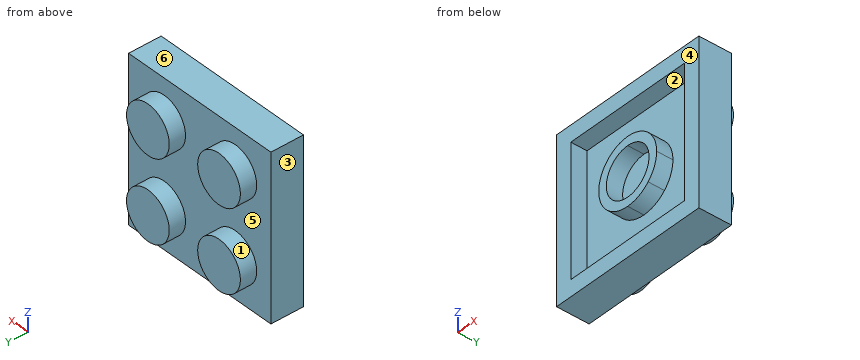
from build123d import *

# Parameters (mm, degrees)
SKETCH1_W           = 2.5
SKETCH1_H           = 1
BOSS_EXTRUDE1_DEPTH = 1
SKETCH1_4_W         = 2.5
SKETCH1_4_H         = 1
BOSS_EXTRUDE3_DEPTH = 1
SKETCH2_R           = 1.5
BOSS_EXTRUDE4_DEPTH = 1


with BuildPart() as part:
    # Sketch1 → Boss-Extrude1 (new body)
    with BuildSketch(Plane(origin=(0, 0, 0), x_dir=(1, 0, 0), z_dir=(0, 1, 0))):
        Polygon((5, 9), (5, 10), (0, 10), (0, 0), (5, 0), (5, 1), (1, 1), (1, 9), align=None)
        with BuildLine():
            Line((5, 7.035533906), (5, 9))
            Line((5, 9), (1, 9))
            Line((1, 9), (1, 1))
            Line((1, 1), (5, 1))
            Line((5, 1), (5, 2.964466094))
            ThreePointArc((5, 2.964466094), (2.964466094, 5), (5, 7.035533906))
        make_face()
        with BuildLine():
            ThreePointArc((6.439339828, 6.439339828), (5.778965102, 6.880588113), (5, 7.035533906))
            Line((5, 7.035533906), (5, 6.5))
            ThreePointArc((5, 6.5), (6.060660172, 6.060660172), (6.5, 5))
            ThreePointArc((6.5, 5), (6.060660172, 3.939339828), (5, 3.5))
            Line((5, 3.5), (5, 2.964466094))
            ThreePointArc((5, 2.964466094), (6.439339828, 3.560660172), (7.035533906, 5))
            ThreePointArc((7.035533906, 5), (6.880588113, 5.778965102), (6.439339828, 6.439339828))
        make_face()
        with BuildLine():
            Line((5, 6.5), (5, 7.035533906))
            ThreePointArc((5, 7.035533906), (2.964466094, 5), (5, 2.964466094))
            Line((5, 2.964466094), (5, 3.5))
            ThreePointArc((5, 3.5), (3.5, 5), (5, 6.5))
        make_face()
        with BuildLine():
            ThreePointArc((6.5, 5), (6.060660172, 6.060660172), (5, 6.5))
            Line((5, 6.5), (5, 3.5))
            ThreePointArc((5, 3.5), (6.060660172, 3.939339828), (6.5, 5))
        make_face()
        with BuildLine():
            Line((5, 3.5), (5, 6.5))
            ThreePointArc((5, 6.5), (3.5, 5), (5, 3.5))
        make_face()
        with BuildLine():
            Line((7.5, 9), (5, 9))
            Line((5, 9), (5, 7.035533906))
            ThreePointArc((5, 7.035533906), (5.778965102, 6.880588113), (6.439339828, 6.439339828))
            ThreePointArc((6.439339828, 6.439339828), (6.114180701, 8.074025149), (7.5, 9))
        make_face()
        with Locations((6.25, 9.5)):
            Rectangle(SKETCH1_W, SKETCH1_H)
        Polygon((10, 10), (7.5, 10), (7.5, 9), (9, 9), (9, 7.5), (10, 7.5), align=None)
        with BuildLine():
            Line((9, 9), (7.5, 9))
            ThreePointArc((7.5, 9), (8.560660172, 8.560660172), (9, 7.5))
            Line((9, 7.5), (9, 9))
        make_face()
        with BuildLine():
            ThreePointArc((9, 7.5), (8.560660172, 8.560660172), (7.5, 9))
            Line((7.5, 9), (7.5, 7.5))
            Line((7.5, 7.5), (9, 7.5))
        make_face()
        with BuildLine():
            Line((7.5, 7.5), (7.5, 9))
            ThreePointArc((7.5, 9), (6.114180701, 8.074025149), (6.439339828, 6.439339828))
            ThreePointArc((6.439339828, 6.439339828), (8.074025149, 6.114180701), (9, 7.5))
            Line((9, 7.5), (7.5, 7.5))
        make_face()
        with BuildLine():
            ThreePointArc((9, 7.5), (8.074025149, 6.114180701), (6.439339828, 6.439339828))
            ThreePointArc((6.439339828, 6.439339828), (6.880588113, 5.778965102), (7.035533906, 5))
            ThreePointArc((7.035533906, 5), (6.439339828, 3.560660172), (5, 2.964466094))
            Line((5, 2.964466094), (5, 1))
            Line((5, 1), (9, 1))
            Line((9, 1), (9, 7.5))
        make_face()
        Polygon((10, 7.5), (9, 7.5), (9, 1), (5, 1), (5, 0), (10, 0), align=None)
    extrude(amount=BOSS_EXTRUDE1_DEPTH)

    # Sketch1_4 → Boss-Extrude3 (add)
    with BuildSketch(Plane(origin=(0, 0, 0), x_dir=(1, 0, 0), z_dir=(0, 1, 0))):
        with BuildLine():
            ThreePointArc((6.439339828, 6.439339828), (5.778965102, 6.880588113), (5, 7.035533906))
            Line((5, 7.035533906), (5, 6.5))
            ThreePointArc((5, 6.5), (6.060660172, 6.060660172), (6.5, 5))
            ThreePointArc((6.5, 5), (6.060660172, 3.939339828), (5, 3.5))
            Line((5, 3.5), (5, 2.964466094))
            ThreePointArc((5, 2.964466094), (6.439339828, 3.560660172), (7.035533906, 5))
            ThreePointArc((7.035533906, 5), (6.880588113, 5.778965102), (6.439339828, 6.439339828))
        make_face()
        with BuildLine():
            Line((5, 6.5), (5, 7.035533906))
            ThreePointArc((5, 7.035533906), (2.964466094, 5), (5, 2.964466094))
            Line((5, 2.964466094), (5, 3.5))
            ThreePointArc((5, 3.5), (3.5, 5), (5, 6.5))
        make_face()
        Polygon((5, 9), (5, 10), (0, 10), (0, 0), (5, 0), (5, 1), (1, 1), (1, 9), align=None)
        Polygon((10, 7.5), (9, 7.5), (9, 1), (5, 1), (5, 0), (10, 0), align=None)
        Polygon((10, 10), (7.5, 10), (7.5, 9), (9, 9), (9, 7.5), (10, 7.5), align=None)
        with Locations((6.25, 9.5)):
            Rectangle(SKETCH1_4_W, SKETCH1_4_H)
    extrude(amount=-BOSS_EXTRUDE3_DEPTH)

    # Sketch2 → Boss-Extrude4 (add)
    with BuildSketch(Plane(origin=(0, 1, 0), x_dir=(1, 0, 0), z_dir=(0, 1, 0))):
        with Locations((7.5, 2.5)):
            Circle(SKETCH2_R)
        with Locations((2.5, 2.5)):
            Circle(SKETCH2_R)
        with Locations((2.5, 7.5)):
            Circle(SKETCH2_R)
        with Locations((7.5, 7.5)):
            Circle(SKETCH2_R)
    extrude(amount=BOSS_EXTRUDE4_DEPTH)


solid = part.part
Model file for the job. Use its own axes, mm. Face numbers are marked on the shaded views. A direction names the side the tool comes from. Give positions to 0.01 mm unless a question says otherwise; leave off trailing zeros. Loops run counter-clockwise (first coordinate to the right, second up) from the corner with the lowest first, then second, coordinate; pieces in that order, holes last.
1) Saw through at D-D (x = 9.5). Write the cut outline in (y, z), plus the area to 3 significant figures.
2) Pull direction Z, two halves, no side cores. Call the marked faces 4, 5 and 6: +Z half, -Z half, draft (parallel to the pull), parting line (faces both ways), or undercut.
3) Saw through at B-B (x = 7.5). Write the cut outline in (y, z).
4) Saw through at A-A (y = -0.2). Write the cut outline in (x, z), plus the area to 3 significant figures.
5) Saw through at C-C (z = -7.5). Write the cut outline in (x, y), plus the area to 3 significant figures.
6) Flat gauge pin, fed straight in: pin 1 Ø1 at (x, z) = (4.5, -5.5) entering from -Y. Where does the tip first touch, or does it go through?
7) Tool access for the marked faces 1, 2 and 3: list every direction of +Z, -Z, +X, -X, +Y, -Y with a clear straight run to the whole face (end or side of a thin tool).
8) Wall check: line 1 (Z direction, x = 5, y = -0.8); line 2 (Z direction, x = 7.5, y = 1.7); line 3 (Z direction, x = 8, y = -0.25). Give the ranges that are in metal, low to high.
Answer block:
1. outline: (-1, -10) - (1, -10) - (1, 0) - (-1, 0) - close
1. area: 20.0 mm2
2. face 4: draft
2. face 5: undercut
2. face 6: +Z half
3. outline: (-1, -10) - (1, -10) - (1, -9) - (2, -9) - (2, -6) - (1, -6) - (1, -4) - (2, -4) - (2, -1) - (1, -1) - (1, 0) - (-1, 0) - (-1, -1) - (0, -1) - (0, -9) - (-1, -9) - close
4. outline: (0, -10) - (10, -10) - (10, 0) - (0, 0) - close; circle Ø4.07 at (5, -5); hole (1, -9) - (9, -9) - (9, -1) - (1, -1) - close; hole circle Ø3 at (5, -5)
4. area: 41.9 mm2
5. outline: (0, -1) - (1, -1) - (1, 0) - (9, 0) - (9, -1) - (10, -1) - (10, 1) - (9, 1) - (9, 2) - (6, 2) - (6, 1) - (4, 1) - (4, 2) - (1, 2) - (1, 1) - (0, 1) - close
5. area: 18.0 mm2
6. pin 1: stops at y = 0
7. face 1: +Y
7. face 2: -Y
7. face 3: +Z, -Z, -X, +Y, -Y
8. line 1: z = -10 to -9, -7.04 to -6.5, -3.5 to -2.96, -1 to 0
8. line 2: z = -9 to -6, -4 to -1
8. line 3: z = -10 to -9, -1 to 0
